Design review of the part built by this model. Coordinates are the model's own, in mm. Coordinates: 2 decimals unless noted, no trailing zeros.
Q1. To check wall thickness, follow probe 1 along X at (y, z) = (1.25, 6.5); probe 2 along Z at (x, y) = (-14, 0.6); probe 3 along Z at (x, y) = (-17, 1.5). State the ranges of each line that lie inside material, in increasing order.
Q2. Clearance check with flat-ended pins moving along their axes: pin 1 Ø1.9 at (x, z) = (24.15, -6.47) entering from +Y; pin 2 Ø1 at (x, y) = (21.5, 1.5) entering from +Z. State where each tip first meets the part, or that it passes through.
Q3. Add section A-A, the plane y = 0.9. Give the number of separate pieces and of enclosed holes in the cut face, plus the area to 3 significant figures.
from build123d import *

# Parameters (mm, degrees)
SKETCH_1_R          = 38
SKETCH_1_R_2        = 22
EXTRUDE_1_DEPTH     = 2
SKETCH_2_R          = 2.1
CUT_EXTRUDE_1_DEPTH = 54.777318639
SKETCH_3_R          = 1.25
CUT_EXTRUDE_2_DEPTH = 54.777318639
SKETCH_5_R          = 1.6
SKETCH_5_R_2        = 2
CUT_EXTRUDE_3_DEPTH = 54.777318639
CUT_EXTRUDE_4_DEPTH = 54.777318639
FILLET_1_R          = 3
EXTRUDE_2_DEPTH     = 2


with BuildPart() as part:
    # 草图1 → 凸台-拉伸1 (new body)
    with BuildSketch(Plane(origin=(0, 0, 0), x_dir=(1, 0, 0), z_dir=(0, 1, 0))):
        with Locations(Location((0, 0, 0), (0, 0, 270))):
            Circle(SKETCH_1_R)
        with Locations(Location((0, 0, 0), (0, 0, 270))):
            Circle(SKETCH_1_R_2, mode=Mode.SUBTRACT)
    extrude(amount=EXTRUDE_1_DEPTH)

    # 草图2 → 切除-拉伸1 (cut, through all)
    with BuildSketch(Plane(origin=(0, 2, 0), x_dir=(1, 0, 0), z_dir=(0, 1, 0))):
        with Locations(Location((13.0112367, 31.411904105, 0), (0, 0, 270))):
            Circle(SKETCH_2_R)
        with Locations(Location((31.411904105, 13.0112367, 0), (0, 0, 270))):
            Circle(SKETCH_2_R)
        with Locations(Location((31.411904105, -13.0112367, 0), (0, 0, 270))):
            Circle(SKETCH_2_R)
        with Locations(Location((13.0112367, -31.411904105, 0), (0, 0, 270))):
            Circle(SKETCH_2_R)
        with Locations(Location((-13.0112367, -31.411904105, 0), (0, 0, 270))):
            Circle(SKETCH_2_R)
        with Locations(Location((-31.411904105, -13.0112367, 0), (0, 0, 270))):
            Circle(SKETCH_2_R)
        with Locations(Location((-31.411904105, 13.0112367, 0), (0, 0, 270))):
            Circle(SKETCH_2_R)
        with Locations(Location((-13.0112367, 31.411904105, 0), (0, 0, 270))):
            Circle(SKETCH_2_R)
    extrude(amount=-CUT_EXTRUDE_1_DEPTH, mode=Mode.SUBTRACT)

    # 草图3 → 切除-拉伸2 (cut, through all)
    with BuildSketch(Plane(origin=(0, 2, 0), x_dir=(1, 0, 0), z_dir=(0, 1, 0))):
        with Locations(Location((12.5, 21.650635095, 0), (0, 0, 270))):
            Circle(SKETCH_3_R)
        with Locations(Location((25, 0, 0), (0, 0, 270))):
            Circle(SKETCH_3_R)
        with Locations(Location((12.5, -21.650635095, 0), (0, 0, 270))):
            Circle(SKETCH_3_R)
        with Locations(Location((-12.5, -21.650635095, 0), (0, 0, 270))):
            Circle(SKETCH_3_R)
        with Locations(Location((-25, 0, 0), (0, 0, 270))):
            Circle(SKETCH_3_R)
        with Locations(Location((-12.5, 21.650635095, 0), (0, 0, 270))):
            Circle(SKETCH_3_R)
    extrude(amount=-CUT_EXTRUDE_2_DEPTH, mode=Mode.SUBTRACT)

    # 草图5 → 切除-拉伸3 (cut, through all)
    with BuildSketch(Plane(origin=(0, 2, 0), x_dir=(1, 0, 0), z_dir=(0, 1, 0))):
        with Locations(Location((24.148145657, 6.470476128, 0), (0, 0, 270))):
            Circle(SKETCH_5_R)
        with Locations(Location((-24.148145657, -6.470476128, 0), (0, 0, 270))):
            Circle(SKETCH_5_R_2)
    extrude(amount=-CUT_EXTRUDE_3_DEPTH, mode=Mode.SUBTRACT)

    # 草图6 → 切除-拉伸4 (cut, through all)
    with BuildSketch(Plane(origin=(0, 2, 0), x_dir=(1, 0, 0), z_dir=(0, 1, 0))):
        with BuildLine():
            Line((-15, 25.980762114), (-19, 32.908965344))
            ThreePointArc((-19, 32.908965344), (-26.870057685, 26.870057685), (-32.908965344, 19))
            Line((-32.908965344, 19), (-25.980762114, 15))
            ThreePointArc((-25.980762114, 15), (-21.213203436, 21.213203436), (-15, 25.980762114))
        make_face()
        with BuildLine():
            ThreePointArc((9.835123714, 36.705181399), (4.959995304, 37.674904732), (0, 38))
            Line((0, 38), (0, 30))
            ThreePointArc((0, 30), (3.915785767, 29.743345841), (7.764571353, 28.977774789))
            Line((7.764571353, 28.977774789), (9.835123714, 36.705181399))
        make_face()
        with BuildLine():
            Line((0, 30), (0, 38))
            ThreePointArc((0, 38), (-4.959995304, 37.674904732), (-9.835123714, 36.705181399))
            Line((-9.835123714, 36.705181399), (-7.764571353, 28.977774789))
            ThreePointArc((-7.764571353, 28.977774789), (-3.915785767, 29.743345841), (0, 30))
        make_face()
        with BuildLine():
            ThreePointArc((32.908965344, 19), (26.870057685, 26.870057685), (19, 32.908965344))
            Line((19, 32.908965344), (15, 25.980762114))
            ThreePointArc((15, 25.980762114), (21.213203436, 21.213203436), (25.980762114, 15))
            Line((25.980762114, 15), (32.908965344, 19))
        make_face()
        with BuildLine():
            Line((36.705181399, 9.835123714), (28.977774789, 7.764571353))
            ThreePointArc((28.977774789, 7.764571353), (29.743345841, 3.915785767), (30, 0))
            ThreePointArc((30, 0), (29.743345841, -3.915785767), (28.977774789, -7.764571353))
            Line((28.977774789, -7.764571353), (36.705181399, -9.835123714))
            ThreePointArc((36.705181399, -9.835123714), (37.674904732, -4.959995304), (38, 0))
            ThreePointArc((38, 0), (37.674904732, 4.959995304), (36.705181399, 9.835123714))
        make_face()
        with BuildLine():
            Line((32.908965344, -19), (25.980762114, -15))
            ThreePointArc((25.980762114, -15), (21.213203436, -21.213203436), (15, -25.980762114))
            Line((15, -25.980762114), (19, -32.908965344))
            ThreePointArc((19, -32.908965344), (26.870057685, -26.870057685), (32.908965344, -19))
        make_face()
        with BuildLine():
            Line((9.835123714, -36.705181399), (7.764571353, -28.977774789))
            ThreePointArc((7.764571353, -28.977774789), (0, -30), (-7.764571353, -28.977774789))
            Line((-7.764571353, -28.977774789), (-9.835123714, -36.705181399))
            ThreePointArc((-9.835123714, -36.705181399), (0, -38), (9.835123714, -36.705181399))
        make_face()
        with BuildLine():
            Line((-19, -32.908965344), (-15, -25.980762114))
            ThreePointArc((-15, -25.980762114), (-21.213203436, -21.213203436), (-25.980762114, -15))
            Line((-25.980762114, -15), (-32.908965344, -19))
            ThreePointArc((-32.908965344, -19), (-26.870057685, -26.870057685), (-19, -32.908965344))
        make_face()
        with BuildLine():
            Line((-36.705181399, -9.835123714), (-28.977774789, -7.764571353))
            ThreePointArc((-28.977774789, -7.764571353), (-30, 0), (-28.977774789, 7.764571353))
            Line((-28.977774789, 7.764571353), (-36.705181399, 9.835123714))
            ThreePointArc((-36.705181399, 9.835123714), (-38, 0), (-36.705181399, -9.835123714))
        make_face()
    extrude(amount=-CUT_EXTRUDE_4_DEPTH, mode=Mode.SUBTRACT)

    # 圆角1
    fillet_1_edges = [part.edges().sort_by_distance(p)[0] for p in [
        (-9.835123714, 1, -36.705181399),
        (9.835123714, 1, -36.705181399),
        (7.764571353, 1, -28.977774789),
        (-7.764571353, 1, -28.977774789),
        (25.980762114, 1, -15),
        (15, 1, -25.980762114),
        (19, 1, -32.908965344),
        (32.908965344, 1, -19),
        (28.977774789, 1, 7.764571353),
        (28.977774789, 1, -7.764571353),
        (36.705181399, 1, -9.835123714),
        (36.705181399, 1, 9.835123714),
        (15, 1, 25.980762114),
        (25.980762114, 1, 15),
        (32.908965344, 1, 19),
        (19, 1, 32.908965344),
        (-7.764571353, 1, 28.977774789),
        (7.764571353, 1, 28.977774789),
        (9.835123714, 1, 36.705181399),
        (-9.835123714, 1, 36.705181399),
        (-25.980762114, 1, 15),
        (-15, 1, 25.980762114),
        (-19, 1, 32.908965344),
        (-32.908965344, 1, 19),
        (-28.977774789, 1, -7.764571353),
        (-28.977774789, 1, 7.764571353),
        (-36.705181399, 1, 9.835123714),
        (-36.705181399, 1, -9.835123714),
        (-15, 1, -25.980762114),
        (-25.980762114, 1, -15),
        (-32.908965344, 1, -19),
        (-19, 1, -32.908965344),
    ]]
    fillet(fillet_1_edges, radius=FILLET_1_R)

    # 草图7 → 凸台-拉伸2 (add)
    with BuildSketch(Plane.XZ):
        with BuildLine():
            Line((22, 0), (20, 0))
            ThreePointArc((20, 0), (18.47759065, -7.653668647), (14.142135624, -14.142135624))
            Line((14.142135624, -14.142135624), (15.556349186, -15.556349186))
            ThreePointArc((15.556349186, -15.556349186), (20.325349715, -8.419035512), (22, 0))
        make_face()
    extrude(amount=-EXTRUDE_2_DEPTH)


solid = part.part
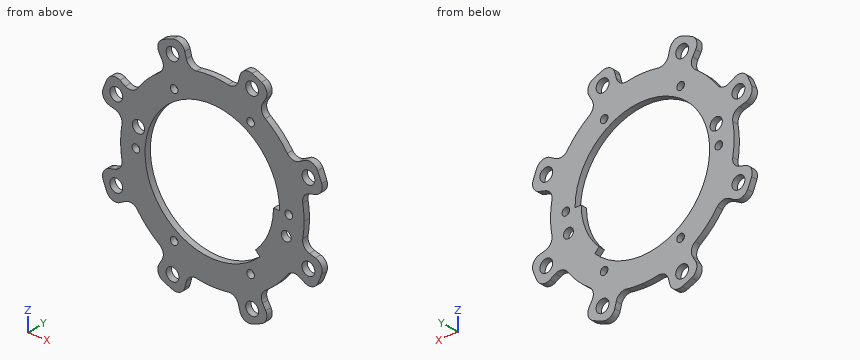
Here are the results:
1. probe 1: x = -29.66 to -26.15, -22.15 to -21.02, 21.02 to 29.66
1. probe 2: z = -35.33 to -33.26, -29.56 to -16.97, 16.97 to 29.56, 33.26 to 35.33
1. probe 3: z = -33.78 to -29.44, -24.75 to -13.96, 13.96 to 24.75, 29.44 to 33.78
2. pin 1: passes through
2. pin 2: stops at z = 21.42
3. separate pieces: 1
3. enclosed holes: 17
3. area: 1,740 mm2
